```python
from build123d import *

# Parameters (mm, degrees)
SKETCH2_R           = 15
BOSS_EXTRUDE1_DEPTH = 10
SKETCH4_W           = 85
SKETCH4_H           = 45
BOSS_EXTRUDE2_DEPTH = 75
CUT_EXTRUDE3_REACH  = 47
SKETCH5_W           = 80
SKETCH5_H           = 70
CUT_EXTRUDE1_REACH  = 87
SKETCH3_R           = 6
SKETCH6_R           = 10
CUT_EXTRUDE4_DEPTH  = 7.5
CUT_EXTRUDE5_REACH  = 87
SKETCH7_R           = 12.5


with BuildPart() as part:
    # Sketch2 → Boss-Extrude1 (new body)
    with BuildSketch(Plane.XY):
        Circle(SKETCH2_R)
    extrude(amount=BOSS_EXTRUDE1_DEPTH)

    # Sketch4 → Boss-Extrude2 (add)
    with BuildSketch(Plane(origin=(0, 0, 0), x_dir=(-1, 0, 0), z_dir=(0, 0, -1))):
        Rectangle(SKETCH4_W, SKETCH4_H)
    extrude(amount=BOSS_EXTRUDE2_DEPTH)

    # Sketch5 → Cut-Extrude3 (cut, up to next)
    with BuildSketch(Plane(origin=(0, 22.5, 0), x_dir=(1, 0, 0), z_dir=(0, 1, 0)), mode=Mode.PRIVATE) as cut_extrude3_sk1:
        with Locations((0, 37.5)):
            Rectangle(SKETCH5_W, SKETCH5_H)
    cut_extrude3_tool1 = extrude(cut_extrude3_sk1.sketch, amount=-CUT_EXTRUDE3_REACH, mode=Mode.PRIVATE) & part.part
    add(cut_extrude3_tool1.solids().sort_by_distance((0, 22.5, -37.5))[0], mode=Mode.SUBTRACT)

    # Sketch3 → Cut-Extrude1 (cut, up to next)
    with BuildSketch(Plane.XY.offset(10), mode=Mode.PRIVATE) as cut_extrude1_sk1:
        Circle(SKETCH3_R)
    cut_extrude1_tool1 = extrude(cut_extrude1_sk1.sketch, amount=-CUT_EXTRUDE1_REACH, mode=Mode.PRIVATE) & part.part
    add(cut_extrude1_tool1.solids().sort_by_distance((0, 0, 10))[0], mode=Mode.SUBTRACT)

    # Sketch6 → Cut-Extrude4 (cut)
    with BuildSketch(Plane(origin=(0, 0, -2.5), x_dir=(-1, 0, 0), z_dir=(0, 0, -1))):
        Circle(SKETCH6_R)
    extrude(amount=-CUT_EXTRUDE4_DEPTH, mode=Mode.SUBTRACT)

    # Sketch7 → Cut-Extrude5 (cut, up to next)
    with BuildSketch(Plane.ZY.offset(42.5), mode=Mode.PRIVATE) as cut_extrude5_sk1:
        with Locations((-37.5, 17.5)):
            Circle(SKETCH7_R)
    cut_extrude5_tool1 = extrude(cut_extrude5_sk1.sketch, amount=-CUT_EXTRUDE5_REACH, mode=Mode.PRIVATE) & part.part
    add(cut_extrude5_tool1.solids().sort_by_distance((-42.5, 17.5, -37.5))[0], mode=Mode.SUBTRACT)


solid = part.part
```
Check sheet for the modelled part. Datum: model origin and axes. Units: mm. A direction names the side the tool comes from. Coordinates: 2 decimals unless noted, no trailing zeros. Order: outer loops, then holes, each group sorted by start corner. A loop starts at its lowest first (then second) coordinate and runs counter-clockwise, first axis right, second up. Notation, with made-up numbers: M 12.5,33 L 62.5,33 A29 ccw 62.5,67 Z; hole C 10,38 d5. An arc over 180 degrees is marked long. Write each question's results on one line, items separated by ' | '. Start each with the question number.
1. Mould release check, pull along Z, two halves, no side actions. Record for faces 6 (the face through (0.6, 15.3, 0)), 7 (the face through (3, 22.5, -73)), 8 (the face through (-41.268, 5.005, -37.847)): +Z half, -Z half, draft (parallel to the pull), parting line (faces both ways), or undercut.
2. Cross-section at C-C on x = -35. Record the cut outline in (y, z).
3. Cross-section at B-B on x = 0. Record the cut outline in (y, z).
4. Cross-section at A-A on z = -37.5. Record the cut outline in (x, y), and give its area (3 significant figures).
5. Material ranges on probe 1 along X at (y, z) = (-19, -66.5); probe 2 along Z at (x, y) = (13, 8.5); probe 3 along Y at (x, z) = (0, 7), recorded low to high.
6. Cross-section at D-D on y = 18. Record the cut outline in (x, z).
7. Access from +Z, -Z, +X, -X, +Y, -Y to the whole of each face (thin tool, end or side, straight path). Record for faces 1 (the face through (-6, 0, 8)), 2 (the face through (42.5, 0, -37)), 3 (the face through (2.17, -9.76, 1.2)), 4 (the face through (-40, 0, -37)), 5 (the face through (6.5, 0.2, 10)).
Checks:
1) face 6: +Z half | face 7: draft | face 8: undercut
2) outline: M -22.5,-75 L 22.5,-75 L 22.5,-72.5 L -22.5,-72.5 Z; M -22.5,-2.5 L 22.5,-2.5 L 22.5,0 L -22.5,0 Z
3) outline: M -22.5,-75 L 22.5,-75 L 22.5,-72.5 L -22.5,-72.5 Z; M -22.5,-2.5 L -10,-2.5 L -10,5 L -6,5 L -6,10 L -15,10 L -15,0 L -22.5,0 Z; M 6,5 L 10,5 L 10,-2.5 L 22.5,-2.5 L 22.5,0 L 15,0 L 15,10 L 6,10 Z
4) outline: M -42.5,-22.5 L -40,-22.5 L -40,5 L -42.5,5 Z; M 40,-22.5 L 42.5,-22.5 L 42.5,22.5 L 40,22.5 Z | area: 181 mm²
5) probe 1: x = -42.5 to -40, 40 to 42.5 | probe 2: z = -75 to -72.5, -2.5 to 0 | probe 3: y = -15 to -6, 6 to 15
6) outline: M -42.5,-75 L 42.5,-75 L 42.5,0 L -42.5,0 L -42.5,-25.01 L -40,-25.01 L -40,-2.5 L 40,-2.5 L 40,-72.5 L -40,-72.5 L -40,-49.99 L -42.5,-49.99 Z
7) face 1: +Z | face 2: +Z, -Z, +X, +Y, -Y | face 3: none | face 4: +Y, -Y | face 5: +Z, +X, -X, +Y, -Y
